The model under review builds one solid part; all positions refer to its coordinate system, in mm. Face numbers are marked on the shaded views. A direction names the side the tool comes from. Coordinates: 2 decimals unless noted, no trailing zeros. Loops run counter-clockwise (first coordinate to the right, second up) from the corner with the lowest first, then second, coordinate; pieces in that order, holes last. Notation, with made-up numbers: M -12.75,6 L -1.75,6 A19 cw -1.75,37 Z; hole C 33,-7.75 d8. An arc over 180 degrees is marked long. Use one line per item in the form item = value.
Autodesk Inventor part; units mm, degrees
ref_plane "YZ Plane" through (0, 0, 0) normal (1, 0, 0) x (0, 1, 0)
ref_plane "XZ Plane" through (0, 0, 0) normal (0, 1, 0) x (-1, 0, 0)
ref_plane "XY Plane" through (0, 0, 0) normal (0, 0, 1) x (1, 0, 0)
sketch "Boceto1" plane through (0, 0, 0) normal (0, 1, 0) x (-1, 0, 0)
  line L0 (-15.2057, -35) -> (14.7943, -35)
  line L1 (14.7943, -35) -> (14.7943, 35)
  line L2 (14.7943, 35) -> (-15.2057, 35)
  line L3 (-15.2057, 35) -> (-15.2057, -35)
  line L4 (-15.2057, -35) -> (14.7943, 35) construction
  line L5 (14.7943, -35) -> (-15.2057, 35) construction
  line L6 (15.2943, 35.5) -> (15.2943, -35.5)
  line L7 (15.2943, -35.5) -> (-15.7057, -35.5)
  line L8 (-15.7057, -35.5) -> (-15.7057, 35.5)
  line L9 (-15.7057, 35.5) -> (15.2943, 35.5)
  line L10 (17.2943, -37.5) -> (17.2943, 37.5)
  line L11 (17.2943, 37.5) -> (-17.7057, 37.5)
  line L12 (-17.7057, 37.5) -> (-17.7057, -37.5)
  line L13 (-17.7057, -37.5) -> (17.2943, -37.5)
  point P0 (0, 0)
  point P1 (-0.2057, 0)
  dimension "d0" = 30
  dimension "d1" = 70
  dimension "d2" = 0.5
  dimension "d3" = 2
extrude "Extrusión1" add sketch "Boceto1" along normal blind 15 contours L13 L12 L11 L10
sketch "Boceto2" plane through (0, 0, 0) normal (0, -1, 0) x (1, 0, 0)
  line L0 (-17.2943, 37.5) -> (17.7057, 37.5)
  line L1 (-17.2943, -37.5) -> (-17.2943, 37.5)
  line L2 (17.7057, -37.5) -> (-17.2943, -37.5)
  line L3 (17.7057, 37.5) -> (17.7057, -37.5)
  line L4 (-15.2943, 35.5) -> (-15.2943, -35.5)
  line L5 (15.7057, 35.5) -> (-15.2943, 35.5)
  line L6 (15.7057, -35.5) -> (15.7057, 35.5)
  line L7 (-15.2943, -35.5) -> (15.7057, -35.5)
  point P0 (0, 0)
extrude "Extrusión2" add sketch "Boceto2" along normal blind 1.5 contours L0 L3 L2 L1 | L5 L6 L7 L4
sketch "Boceto3" plane through (0, -1.5, 0) normal (0, -1, 0) x (1, 0, 0)
  line L0 (-17.2943, -37.5) -> (17.7057, -37.5)
  line L1 (17.7057, -37.5) -> (17.7057, 37.5)
  line L2 (17.7057, 37.5) -> (-17.2943, 37.5)
  line L3 (-17.2943, 37.5) -> (-17.2943, -37.5)
  line L4 (-17.2943, 37.5) -> (17.7057, 37.5)
  line L5 (17.7057, 37.5) -> (17.7057, 44.5)
  line L6 (17.7057, 44.5) -> (-17.2943, 44.5)
  line L7 (-17.2943, 44.5) -> (-17.2943, 37.5)
  circle A0 centre (0.2057, 41) radius 1.5
  arc A1 (3.6377, 40.3136) -> (-3.2839, 40.7308) centre (0.2057, 41) ccw
  arc A2 (-3.5482, 41.7508) -> (-3.2839, 40.7308) centre (-6.2751, 40.5) ccw
  arc A3 (3.6953, 40.7308) -> (6.6864, 37.5) centre (6.6864, 40.5) ccw
  line L8 (3.6377, 40.3136) -> (17.7057, 37.5)
  line L9 (-17.2943, 44.5) -> (-3.2263, 41.6864)
  line L10 (-1.2652, 41.2942) -> (1.6766, 40.7058)
  point P0 (0, 0)
  point P1 (3.6929, 40.3026)
  point P2 (-6.2751, 37.5)
  dimension "d8" = 7
  dimension "d9" = 35
  dimension "d10" = 3
  dimension "d11" = 6
  dimension "d12" = 6
  dimension "d13" = 7
extrude "Extrusión3" add sketch "Boceto3" against normal blind 1.5 contours A2 A1 L8 A3 L2
mirror "Simetría1" about plane through (0, 0, 0) normal (0, 0, 1) of "Extrusión3"
sketch "Boceto4" plane through (-15.2943, 15, 35.5) normal (1, 0, 0) x (0, 0, -1)
  line L0 (0, -15) -> (71, -15)
  line L1 (71, -15) -> (71, 0)
  line L2 (0, 0) -> (71, 0)
  line L3 (0, -15) -> (0, 0)
  line L4 (0, -15) -> (30, -15)
  line L5 (30, -15) -> (30, -12)
  line L6 (30, -12) -> (18, -12)
  line L7 (18, -12) -> (30, -12)
  line L8 (30, -12) -> (30, -8)
  line L9 (30, -8) -> (18, -8)
  line L10 (18, -8) -> (18, -12)
  point P0 (35.5, -15)
  dimension "d16" = 30
  dimension "d17" = 3
  dimension "d18" = 12
extrude "Extrusión4" cut sketch "Boceto4" against normal up to surface (2 mm away) contours L6 L10 L9 L8
sketch "Boceto5" plane through (15.7057, 15, -35.5) normal (-1, 0, 0) x (0, 0, 1)
  line L0 (71, -15) -> (71, 0)
  line L1 (71, 0) -> (17, 0)
  line L2 (0, 0) -> (71, 0)
  line L3 (71, -15) -> (17, -15)
  line L4 (0, -15) -> (71, -15)
  line L5 (17, -15) -> (17, -10)
  line L6 (17, -10) -> (17, 0)
  line L7 (17, -10) -> (35, -10)
  line L8 (35, -10) -> (35, 0)
  line L9 (35, 0) -> (17, 0)
  line L10 (17, 0) -> (17, -10)
  point P0 (35.5, -15)
  point P1 (17, 0)
  dimension "d21" = 54
  dimension "d22" = 54
  dimension "d23" = 5
  dimension "d24" = 10
  dimension "d25" = 18
  dimension "d26" = 10
extrude "Extrusión5" cut sketch "Boceto5" against normal blind 10 contours L8 L7 L6 L1
properties part number "Caja"
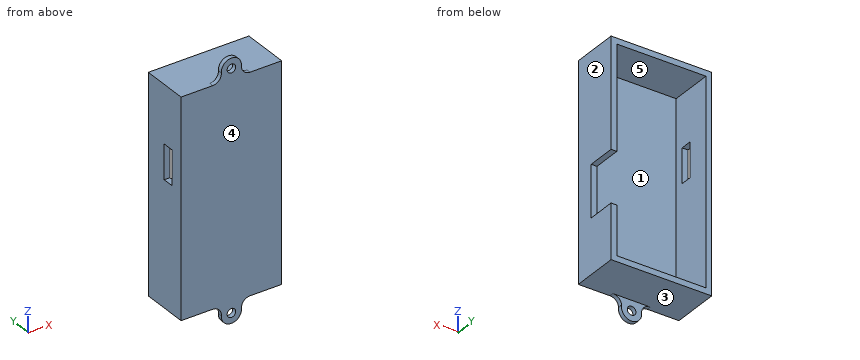
1. Insertion check: P1, Ø8, axis at x = 9.5, y = 1.5, coming from the +Z side; P2, Ø12, axis at x = -6, z = -22.5, coming from the +Y side; P3, Ø3, axis at x = -1.5, y = 13, coming from the -Z side. Each pin has a flat end and moves straight along its axis. Give the tip position at first contact, or say it passes through.
Response values:
P1 = 37.64
P2 = 0
P3 = -37.5
2. The part is to be moulded in two halves that separate along X. For the marked faces 1, 2 and 3, say which applies: pulls with the +X half, pulls with the -X half, needs draft (parallel to the pull), parting line crosses it, or undercut.
Response values:
face_1 = undercut
face_2 = pulls with the +X half
face_3 = needs draft
3. Add section D-D (x = 2.5). State the section outline as (y, z) points, then the cut area to 3 significant figures.
Response values:
outline = M -1.5,-43.64 L 0,-43.64 L 0,-37.5 L 15,-37.5 L 15,-35.5 L 0,-35.5 L 0,35.5 L 15,35.5 L 15,37.5 L 0,37.5 L 0,43.64 L -1.5,43.64 Z
area = 191 mm^2
4. Add section C-C (y = 11.5). State the section outline as (x, z) points, then the cut area to 3 significant figures.
Response values:
outline = M -17.29,-37.5 L 17.71,-37.5 L 17.71,-18.5 L 15.71,-18.5 L 15.71,-35.5 L -15.29,-35.5 L -15.29,35.5 L 15.71,35.5 L 15.71,-0.5 L 17.71,-0.5 L 17.71,37.5 L -17.29,37.5 Z
area = 388 mm^2
5. Wall thickness on line 1 along X through (y, z) = (-0.85, 41); line 2 along Z through (x, y) = (-7, 12); line 3 along X through (y, z) = (1, 5.5): over which ranges is each line inside the solid? List them lowest first. Write a range as from..to.
Response values:
line_1 = -3.29..-1.29, 1.71..3.71
line_2 = -37.5..-35.5, 35.5..37.5
line_3 = -17.29..-15.29, 15.71..17.71
6. Machinability: for the marked faces 4 and 5, which of the approach directions +Z, -Z, +X, -X, +Y, -Y give a long, thin tool a straight path to every point of the face, cutting with its end or side? Answer none if there is none.
Response values:
face_4 = +Z, -Z, +X, -X, -Y
face_5 = +Y
7. Add section A-A (x = 11). State the section outline as (y, z) points.
Response values:
outline = M -1.5,-37.5 L 15,-37.5 L 15,-35.5 L 0,-35.5 L 0,35.5 L 15,35.5 L 15,37.5 L -1.5,37.5 Z
8. Add section B-B (z = -13). State the section outline as (x, y) points, then the cut area to 3 significant figures.
Response values:
outline = M -17.29,-1.5 L 17.71,-1.5 L 17.71,5 L 15.71,5 L 15.71,0 L -15.29,0 L -15.29,15 L -17.29,15 Z
area = 92.5 mm^2
